Geometry check sheet. Reference: the model listing, model coordinates, mm. A direction names the side the tool comes from. Coordinates: 2 decimals unless noted, no trailing zeros. Write each loop counter-clockwise with the first axis right and the second up, starting at its lowest first coordinate (ties: lowest second). Pieces come first, ordered by that corner, then holes. Notation, with made-up numbers: (4, 43) -> (31, 43) arc R28 cw to (31, 81) -> close; hole circle Ø9 at (-16, 64). An arc over 180 degrees is marked (long way). Answer as CSV lines item,"result".
Autodesk Fusion 360 part; units mm, degrees
sketch "Sketch1" plane through (0, 0, 0) normal (0, 0, 1) x (1, 0, 0)
  line L0 (36.125, -21.42) -> (-36.125, -21.42)
  line L1 (-36.125, -21.42) -> (-36.125, 21.42)
  line L2 (-36.125, 21.42) -> (36.125, 21.42)
  line L3 (36.125, 21.42) -> (36.125, -21.42)
  line L4 (36.125, -21.42) -> (-36.125, 21.42) construction
  line L5 (-36.125, -21.42) -> (36.125, 21.42) construction
  line L6 (31.15, -20) -> (-31.15, -20)
  line L7 (-31.15, -20) -> (-31.15, 20)
  line L8 (-31.15, 20) -> (31.15, 20)
  line L9 (31.15, 20) -> (31.15, -20)
  line L10 (31.15, -20) -> (-31.15, 20) construction
  line L11 (-31.15, -20) -> (31.15, 20) construction
  line L12 (28.75, -15) -> (-28.75, 15) construction
  line L13 (-28.75, -15) -> (28.75, 15) construction
  line L14 (36.125, -18.0538) -> (34.125, -18.0538) construction
  line L15 (34.125, -21.42) -> (34.125, 22) construction
  line L16 (-36.125, 20.5191) -> (-34.125, 20.5191) construction
  line L17 (-34.125, 20.5191) -> (-34.125, -21.42) construction
  circle A0 centre (-34.125, -19.236) radius 1.2
  line L18 (-34.125, -21.42) -> (-34.125, -20.67)
  line L19 (-34.1139, 21.42) -> (-34.1139, 19.27) construction
  circle A1 centre (-34.1139, 19.27) radius 1.2
  line L20 (34.125, 21.42) -> (34.125, 19.27) construction
  circle A2 centre (34.125, 19.27) radius 1.2
  line L21 (34.125, -21.42) -> (34.125, -19.27) construction
  circle A3 centre (34.125, -19.27) radius 1.2
  line L22 (0, 21.42) -> (0, 17.42) construction
  line L23 (0, 17.42) -> (28.75, 17.42) construction
  line L24 (28.75, 17.42) -> (-28.75, 17.42)
  line L25 (-28.75, 17.42) -> (-28.75, -12.58)
  line L26 (-28.75, -12.58) -> (28.75, -12.58)
  line L27 (28.75, -12.58) -> (28.75, 17.42)
  circle A4 centre (34.125, 19.27) radius 2
  circle A5 centre (-34.1139, 19.27) radius 2
  circle A6 centre (-34.125, -19.236) radius 2
  circle A7 centre (34.125, -19.27) radius 2
  line L28 (38.125, 23.42) -> (-38.125, 23.42)
  line L29 (-38.125, 23.42) -> (-38.125, -23.42)
  line L30 (-38.125, -23.42) -> (38.125, -23.42)
  line L31 (38.125, -23.42) -> (38.125, 23.42)
  line L32 (38.125, 23.42) -> (-38.125, -23.42) construction
  line L33 (-38.125, 23.42) -> (38.125, -23.42) construction
  line L34 (37.25, 22.25) -> (-37.25, 22.25)
  line L35 (-37.25, 22.25) -> (-37.25, -22.25)
  line L36 (-37.25, -22.25) -> (37.25, -22.25)
  line L37 (37.25, -22.25) -> (37.25, 22.25)
  line L38 (37.25, 22.25) -> (-37.25, -22.25) construction
  line L39 (-37.25, 22.25) -> (37.25, -22.25) construction
  dimension "d1" = 72.25
  dimension "d2" = 42.84
  dimension "d3" = 62.3
  dimension "d4" = 40
  dimension "d5" = 57.5
  dimension "d6" = 30
  dimension "d7" = 2
  dimension "d8" = 2
  dimension "d9" = 2.4
  dimension "d11" = 0.75
  dimension "d12" = 2.15
  dimension "d13" = 2.4
  dimension "d14" = 2.4
  dimension "d15" = 2.15
  dimension "d16" = 2.4
  dimension "d17" = 2.15
  dimension "d18" = 2.4
  dimension "d19" = 4
  dimension "d20" = 28.75
  dimension "d21" = 57.5
  dimension "d22" = 30
  dimension "d24" = 30
  dimension "d27" = 30
  dimension "d28" = 4
  dimension "d29" = 4
  dimension "d30" = 4
  dimension "d31" = 4
  dimension "d37" = 76.25
  dimension "d38" = 46.84
  dimension "d39" = 74.5
  dimension "d40" = 44.5
extrude "Extrude1" add sketch "Sketch1" against normal blind 3.1 contours A7 | A4 | A6 | A5 makes body 1 at (36.1225, 19.1703, -2.0667) makes body 2 at (36.1225, -19.3697, -2.0667) makes body 3 at (-32.1164, 19.1703, -2.0667) makes body 4 at (-32.1349, -19.0369, -1.0333)
extrude "Extrude2" add sketch "Sketch1" along normal blind 1 contours A7 | A4 | L0 L1 L2 L3 L18 A6 | L0 L1 L18 A6 | A6 | L6 L7 L8 L9 | A0 | A1 | A2 | A3 | A5 | L28 L29 L30 L31 | L34 L35 L36 L37 bodies 1 2 3 4
extrude "Extrude3" add sketch "Sketch1" against normal blind 3 contours L34 L35 L36 L37 bodies 1
fillet "Fillet1" radius 1 4 edges at (-38.125, 0, 1) (0, -23.42, 1) (38.125, 0, 1) (0, 23.42, 1) on bodies 1
chamfer "Chamfer1" distance 3 distance2 0.9 4 edges at (28.75, 2.42, 1) (0, 17.42, 1) (-28.75, 2.42, 1) (0, -12.58, 1) measured on face at (9.5833, -19.1401, 1) measured on face at (9.5833, -19.1401, 1) measured on face at (9.5833, -19.1401, 1) measured on face at (9.5833, -19.1401, 1) on bodies 1
sketch "Sketch2" plane through (0, 0, -3.1) normal (0, 0, -1) x (1, 0, 0)
  circle A0 centre (-34.125, 19.236) radius 1.2
  circle A1 centre (-34.125, 19.236) radius 2
  line L0 (-36.1253, 21.4221) -> (36.1242, 21.4221)
  line L1 (36.1242, 21.4221) -> (36.1242, -21.4189)
  line L2 (36.1242, -21.4189) -> (-36.1253, -21.4189)
  line L3 (-36.1253, -21.4189) -> (-36.1253, 21.4221)
  line L4 (-31.15, -20) -> (31.15, -20)
  line L5 (31.15, -20) -> (31.15, 20)
  line L6 (31.15, 20) -> (-31.15, 20)
  line L7 (-31.15, 20) -> (-31.15, -20)
  circle A2 centre (34.1232, 19.2725) radius 1.2039
  circle A3 centre (-34.125, 19.236) radius 1.2
  circle A4 centre (-34.1138, -19.2699) radius 1.1936
  circle A5 centre (34.1249, -19.2699) radius 1.194
  line L8 (-28.7509, 12.58) -> (28.75, 12.58)
  line L9 (28.75, 12.58) -> (28.75, -17.42)
  line L10 (28.75, -17.42) -> (-28.7509, -17.42)
  line L11 (-28.7509, -17.42) -> (-28.7509, 12.58)
extrude "Extrude1'" add sketch "Sketch2" against normal blind 1.12 separate body contours L0 L1 L2 L3 | L4 L5 L6 L7 | L8 L9 L10 L11 makes body 5 in component "Component"
extrude "Extrude2'" add sketch "Sketch2" against normal blind 3 contours L4 L5 L6 L7 bodies 5 in component "Component"
extrude "Extrude3'" add sketch "Sketch2" against normal blind 2.5 contours L8 L9 L10 L11 bodies 5 in component "Component"
extrude "Extrude4" add sketch "Sketch2" against normal blind 1.12 contours A1 bodies 5 in component "Component"
component "Component" placed x (1, 0, 0) y (0, 1, 0) z (0, 0, 1) at (0, 0, 0)
hidden bodies 1
equation "d20 = ( 57.5 / 2 ) * 1 mm"
Item 1: Thickness scan on probe 1 along X at (y, z) = (-12, -0.3); probe 2 along X at (y, z) = (12.5, -1.4); probe 3 along Z at (x, y) = (32.5, -10). Record the ranges inside material, lowest first.
Responses:
probe 1,"x = -31.15 to -28.75, 28.75 to 31.15"
probe 2,"x = -31.15 to 31.15"
probe 3,"z = -3.1 to -1.98"
Item 2: Cross-section at A-A, the plane y = 2.5. Record the cut outline in (x, z), plus the area to 3 significant figures.
Responses:
outline,"(-36.13, -3.1) -> (36.12, -3.1) -> (36.12, -1.98) -> (31.15, -1.98) -> (31.15, -0.1) -> (28.75, -0.1) -> (28.75, -0.6) -> (-28.75, -0.6) -> (-28.75, -0.1) -> (-31.15, -0.1) -> (-31.15, -1.98) -> (-36.13, -1.98) -> close"
area,"169 mm2"
Item 3: Release check for a two-part mould opening along X. For faces 4 (the cylindrical face through (35.264, 18.911, -2.548)), 5 (the flat face through (31.15, 0, -1)), 6 (the flat face through (0, -20, -1)) record: +X half, -X half, draft (parallel to the pull), parting line (faces both ways), or undercut.
Responses:
face 4,"undercut"
face 5,"+X half"
face 6,"draft"
Item 4: Depth check by flat-ended pin: pin 1 Ø0.6 at (x, z) = (-6.5, -1.5) entering from +Y; pin 2 Ø3 at (x, y) = (34.12, -19.27) entering from -Z; pin 3 Ø9 at (x, y) = (-10.5, 0) entering from +Z; pin 4 Ø0.6 at (y, z) = (1, -0.5) entering from -X. Enter the tip coordinate at first touch or a pass-through.
Responses:
pin 1,"stops at y = 20"
pin 2,"stops at z = -3.1"
pin 3,"stops at z = -0.6"
pin 4,"stops at x = -31.15"
Item 5: Cross-section at B-B, the plane x = -1.5. Record the cut outline in (y, z), plus the area to 3 significant figures.
Responses:
outline,"(-21.42, -3.1) -> (21.42, -3.1) -> (21.42, -1.98) -> (20, -1.98) -> (20, -0.1) -> (17.42, -0.1) -> (17.42, -0.6) -> (-12.58, -0.6) -> (-12.58, -0.1) -> (-20, -0.1) -> (-20, -1.98) -> (-21.42, -1.98) -> close"
area,"108 mm2"
Item 6: Set-up check for faces 1 (the flat face through (-31.15, 0, -1)), 2 (the flat face through (0, 2, -0.6)), 3 (the flat face through (0, 20, -1)): record each of +Z, -Z, +X, -X, +Y, -Y from which the full face is reachable in a straight line by a thin tool's end or side.
Responses:
face 1,"+Z, -X, +Y, -Y"
face 2,"+Z"
face 3,"+Z, +X, -X, +Y"
Item 7: Cross-section at C-C, the plane z = -1.1. Record the cut outline in (x, y), plus the area to 3 significant figures.
Responses:
outline,"(-31.15, -20) -> (31.15, -20) -> (31.15, 20) -> (-31.15, 20) -> close"
area,"2,490 mm2"
Item 8: Cross-section at D-D, the plane x = -29.5. Record the cut outline in (y, z), plus the area to 3 significant figures.
Responses:
outline,"(-21.42, -3.1) -> (21.42, -3.1) -> (21.42, -1.98) -> (20, -1.98) -> (20, -0.1) -> (-20, -0.1) -> (-20, -1.98) -> (-21.42, -1.98) -> close"
area,"123 mm2"
